from build123d import *

# Parameters (mm, degrees)
SKETCH1_R           = 20
BOSS_EXTRUDE1_DEPTH = 20
SKETCH4_W           = 5
SKETCH4_H           = 2.912778991
SKETCH5_R           = 3.055550827
CUT_EXTRUDE2_DEPTH  = 35.641016151


with BuildPart() as part:
    # Sketch1 → Boss-Extrude1 (new body)
    with BuildSketch(Plane.XY):
        Circle(SKETCH1_R)
    extrude(amount=BOSS_EXTRUDE1_DEPTH)

    # Sketch4 → Cut-Revolve1 (revolve, cut)
    with BuildSketch(Plane(origin=(0, 0, 0), x_dir=(0, 0, -1), z_dir=(1, 0, 0)), mode=Mode.PRIVATE) as cut_revolve1_sk:
        with Locations((-10, 19.456389495)):
            Rectangle(SKETCH4_W, SKETCH4_H)
    revolve(cut_revolve1_sk.sketch.rotate(Axis((0, 0, 0), (0, 0, 1)), 90), axis=Axis((0, 0, 0), (0, 0, 1)), mode=Mode.SUBTRACT)

    # Sketch5 → Cut-Extrude2 (cut, through all)
    with BuildSketch(Plane(origin=(0, 0, 0), x_dir=(-1, 0, 0), z_dir=(0, 0, -1))):
        with Locations((-12.052497778, -4.218156491)):
            Circle(SKETCH5_R)
    extrude(amount=-CUT_EXTRUDE2_DEPTH, mode=Mode.SUBTRACT)


solid = part.part
Verification items for the finished model (mm, model axes). A direction names the side the tool comes from. Coordinates: 2 decimals unless noted, no trailing zeros. Loops run counter-clockwise (first coordinate to the right, second up) from the corner with the lowest first, then second, coordinate; pieces in that order, holes last. Notation, with made-up numbers: (80.25, 26.5) -> (93.25, 26.5) arc R17 ccw to (93.25, 49.5) -> close; hole circle Ø1 at (63, 34). An arc over 180 degrees is marked (long way). Answer as a JSON object with one key per item and string values. Group by question number.
Item 1: Depth check by flat-ended pin: pin 1 (6 mm diameter, centred on x = 2.5, z = 7.5, fed in from +Y); pin 2 (3 mm diameter, centred on x = 14, z = 13, fed in from +Y); pin 3 (5 mm diameter, centred on x = -3.5, z = 11, fed in from -Y). Enter the tip coordinate at first touch or a pass-through.
Item 2: Mould release check, pull along Z, two halves, no side actions. Record for faces 1 (the flat face through (0, 0, 0)), 2 (the flat face through (-18, -3, 12.5)), 3 (the cylindrical face through (9.23, -5.39, 9.86)): +Z half, -Z half, draft (parallel to the pull), parting line (faces both ways), or undercut.
Item 3: Sectioned sample at C-C on x = 14.5. Record the boundary of the cut face in (y, z).
Item 4: Sectioned sample at A-A on x = 0. Record the boundary of the cut face in (y, z).
Item 5: Sectioned sample at D-D on y = 17. Record the boundary of the cut face in (x, z), plus the area to 3 significant figures.
Item 6: Tool access check on faces 4 (the flat face through (-18, -3, 7.5)), 5 (the cylindrical face through (-4.336, -19.524, 3.698)). Record the directions out of +Z, -Z, +X, -X, +Y, -Y that give a thin tool (end or side, any length) a straight path to the whole face; none if there is none.
Item 7: Sectioned sample at B-B on y = -2. Record the boundary of the cut face in (x, z).
Item 8: Scan lines: probe 1 along Y at (x, z) = (11, 11); probe 2 along X at (y, z) = (13, 9.5); probe 3 along Y at (x, z) = (-11.5, 14). Record each from-to range of solid material in increasing order.
Evaluation:
{
 "1": {"pin 1": "stops at y = 20", "pin 2": "stops at y = 15.61", "pin 3": "stops at y = -19.94"},
 "2": {"face 1": "-Z half", "face 2": "undercut", "face 3": "draft"},
 "3": {"outline": "(-13.77, 0) -> (-6.05, 0) -> (-6.05, 20) -> (-13.77, 20) -> (-13.77, 12.5) -> (-10.67, 12.5) -> (-10.67, 7.5) -> (-13.77, 7.5) -> close; (-2.39, 0) -> (13.77, 0) -> (13.77, 7.5) -> (10.67, 7.5) -> (10.67, 12.5) -> (13.77, 12.5) -> (13.77, 20) -> (-2.39, 20) -> close"},
 "4": {"outline": "(-20, 0) -> (20, 0) -> (20, 7.5) -> (18, 7.5) -> (18, 12.5) -> (20, 12.5) -> (20, 20) -> (-20, 20) -> (-20, 12.5) -> (-18, 12.5) -> (-18, 7.5) -> (-20, 7.5) -> close"},
 "5": {"outline": "(-10.54, 0) -> (10.54, 0) -> (10.54, 7.5) -> (5.92, 7.5) -> (5.92, 12.5) -> (10.54, 12.5) -> (10.54, 20) -> (-10.54, 20) -> (-10.54, 12.5) -> (-5.92, 12.5) -> (-5.92, 7.5) -> (-10.54, 7.5) -> close", "area": "375 mm²"},
 "6": {"face 4": "none", "face 5": "+Z, -Z"},
 "7": {"outline": "(-19.9, 0) -> (9.95, 0) -> (9.95, 20) -> (-19.9, 20) -> (-19.9, 12.5) -> (-17.89, 12.5) -> (-17.89, 7.5) -> (-19.9, 7.5) -> close; (14.15, 0) -> (19.9, 0) -> (19.9, 7.5) -> (17.89, 7.5) -> (17.89, 12.5) -> (19.9, 12.5) -> (19.9, 20) -> (14.15, 20) -> close"},
 "8": {"probe 1": "y = -14.25 to -7.09, -1.35 to 14.25", "probe 2": "x = -12.45 to 12.45", "probe 3": "y = -16.36 to 16.36"}
}
